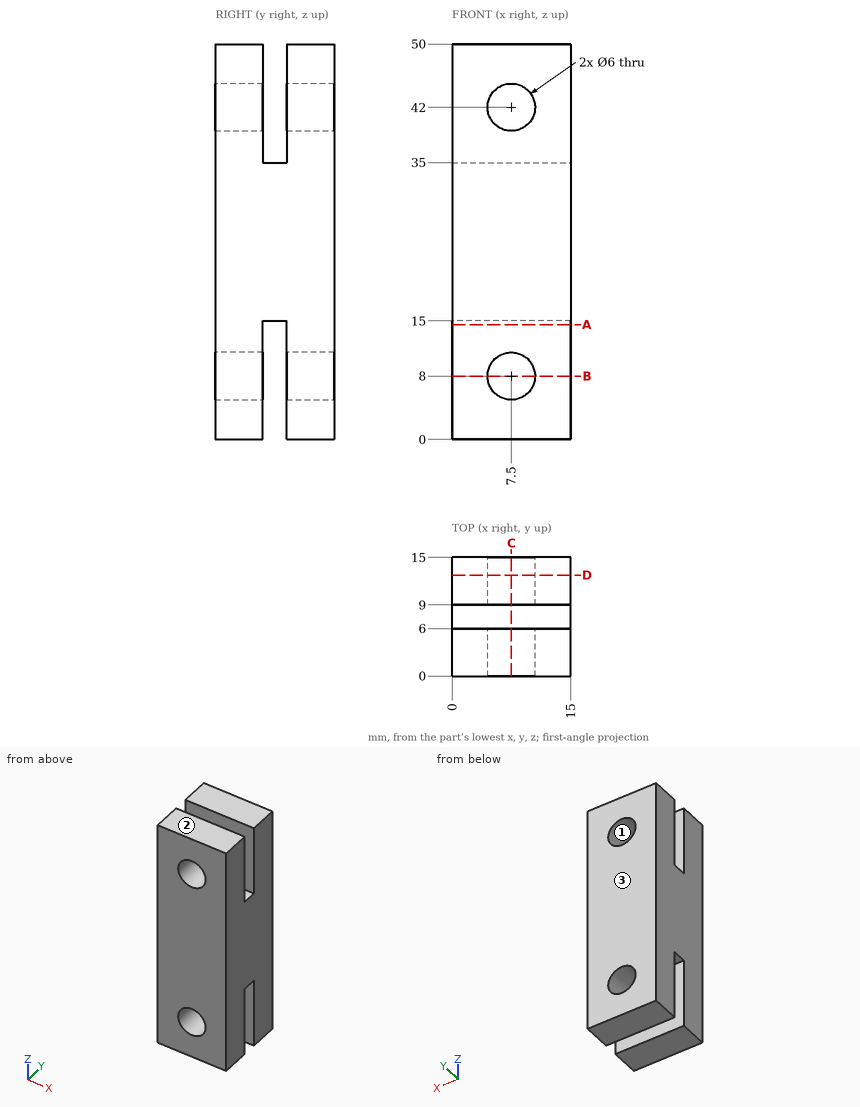
For this review, use the dimensioned drawing (mm, ordinates from the lowest corner) and the shaded views. Round coordinates to 2 decimals unless told otherwise and drop trailing zeros. Loops run counter-clockwise (first coordinate to the right, second up) from the corner with the lowest first, then second, coordinate; pieces in that order, holes last. Notation, with made-up numbers: (-11.75, -32.75) -> (47.25, -32.75) arc R10 ccw to (47.25, -23.75) -> close; hole circle Ø1 at (57, -29.75). An arc over 180 degrees is marked (long way). Write item = value, one per line. Start each with the question number.
Item 1: Take a section at D-D on y = 12.75. Give the boundary of the cut face in (x, z), plus the area to 3 significant figures.
Item 2: Take a section at B-B on z = 8. Give the boundary of the cut face in (x, y), plus the area to 3 significant figures.
Item 3: To check wall thickness, follow L1, parallel to Z at x = 7.75, y = 10; L2, parallel to X at y = 12.85, z = 42; L3, parallel to Z at x = 8.25, y = 14. State the ranges of each line that lie inside material, in increasing order.
Item 4: Take a section at A-A on z = 14.5. Give the boundary of the cut face in (x, y), plus the area to 3 significant figures.
Item 5: Take a section at C-C on x = 7.5. Give the boundary of the cut face in (y, z).
Item 6: Mouldability with a two-part tool opening along Z and no side actions: class the marked faces 1, 2 and 3 as released by +Z, released by -Z, zero draft, split by the parting line, or undercut.
Result:
q1.outline = (0, 0) -> (15, 0) -> (15, 50) -> (0, 50) -> close; hole circle Ø6 at (7.5, 8); hole circle Ø6 at (7.5, 42)
q1.area = 693 mm²
q2.outline = (0, 0) -> (4.5, 0) -> (4.5, 6) -> (0, 6) -> close; (0, 9) -> (4.5, 9) -> (4.5, 15) -> (0, 15) -> close; (10.5, 0) -> (15, 0) -> (15, 6) -> (10.5, 6) -> close; (10.5, 9) -> (15, 9) -> (15, 15) -> (10.5, 15) -> close
q2.area = 108 mm²
q3.L1 = 0 to 5.01, 10.99 to 39.01, 44.99 to 50
q3.L2 = 0 to 4.5, 10.5 to 15
q3.L3 = 0 to 5.1, 10.9 to 39.1, 44.9 to 50
q4.outline = (0, 0) -> (15, 0) -> (15, 6) -> (0, 6) -> close; (0, 9) -> (15, 9) -> (15, 15) -> (0, 15) -> close
q4.area = 180 mm²
q5.outline = (0, 0) -> (6, 0) -> (6, 5) -> (0, 5) -> close; (0, 11) -> (6, 11) -> (6, 15) -> (9, 15) -> (9, 11) -> (15, 11) -> (15, 39) -> (9, 39) -> (9, 35) -> (6, 35) -> (6, 39) -> (0, 39) -> close; (0, 45) -> (6, 45) -> (6, 50) -> (0, 50) -> close; (9, 0) -> (15, 0) -> (15, 5) -> (9, 5) -> close; (9, 45) -> (15, 45) -> (15, 50) -> (9, 50) -> close
q6.face_1 = undercut
q6.face_2 = released by +Z
q6.face_3 = zero draft
